Drawing for the job (mm, zero at the part's lowest x, y, z). A direction names the side the tool comes from. Round coordinates to 2 decimals unless told otherwise and drop trailing zeros. Order: outer loops, then holes, each group sorted by start corner. A loop starts at its lowest first (then second) coordinate and runs counter-clockwise, first axis right, second up. Notation, with made-up numbers: M 7.5,21.5 L 16.5,21.5 A19 cw 16.5,34.5 Z; hole C 81,74.25 d3. An arc over 180 degrees is marked long. Answer as CSV lines item,"result". Start each with the question number.
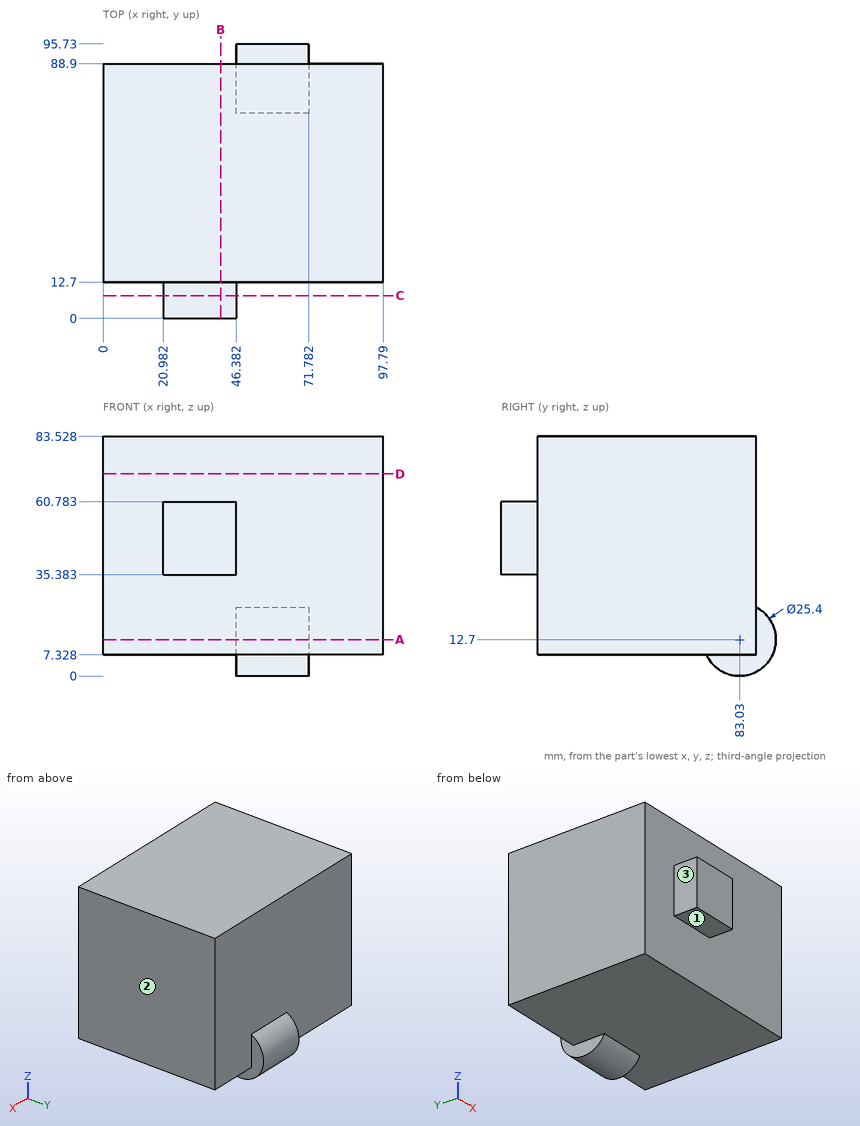
Q1. Band-saw the part on C-C, the plane y = 8. Write the cut outline in (x, z).
Q2. Drop flat-ended pins along their axis: P1, Ø4, axis at x = 19.5, z = 67.5, coming from the -Y side; P2, Ø6.5, axis at y = 5.5, z = 46.5, coming from the -X side; P3, Ø12, axis at x = 39, z = 40.5, coming from the +Y side. Give the stop position or say it passes through.
Q3. Band-saw the part on B-B, the plane x = 41. Write the cut outline in (y, z), then the cut area to 3 significant figures.
Q4. Band-saw the part on D-D, the plane z = 70.5. Write the cut outline in (x, y).
Q5. Band-saw the part on A-A, the plane z = 12.7. Write the cut outline in (x, y), then the cut area to 4 significant figures.
Q6. Probe line 1 along Z through (x, y) = (47, 42.5); line 2 along Y through (x, z) = (62.5, 48.5); line 3 along Y through (x, z) = (21.5, 49). List the from-to ranges inside material, lowest first. Write a range as from..to.
Q7. Tool access for the marked faces 1, 2 and 3: list every direction of +Z, -Z, +X, -X, +Y, -Y with a clear straight run to the whole face (end or side of a thin tool).
Answer:
1,outline,"M 20.98,35.38 L 46.38,35.38 L 46.38,60.78 L 20.98,60.78 Z"
2,P1,"stops at y = 12.7"
2,P2,"stops at x = 20.98"
2,P3,"stops at y = 88.9"
3,outline,"M 0,35.38 L 12.7,35.38 L 12.7,7.33 L 88.9,7.33 L 88.9,83.53 L 12.7,83.53 L 12.7,60.78 L 0,60.78 Z"
3,area,"6,130 mm^2"
4,outline,"M 0,12.7 L 97.79,12.7 L 97.79,88.9 L 0,88.9 Z"
5,outline,"M 0,12.7 L 97.79,12.7 L 97.79,88.9 L 71.78,88.9 L 71.78,95.73 L 46.38,95.73 L 46.38,88.9 L 0,88.9 Z"
5,area,"7,625 mm^2"
6,line 1,"z = 7.33..83.53"
6,line 2,"y = 12.7..88.9"
6,line 3,"y = 0..88.9"
7,face 1,"-Z, +X, -X, -Y"
7,face 2,"+Z, -Z, +X, +Y, -Y"
7,face 3,"+Z, -Z, -X, -Y"
